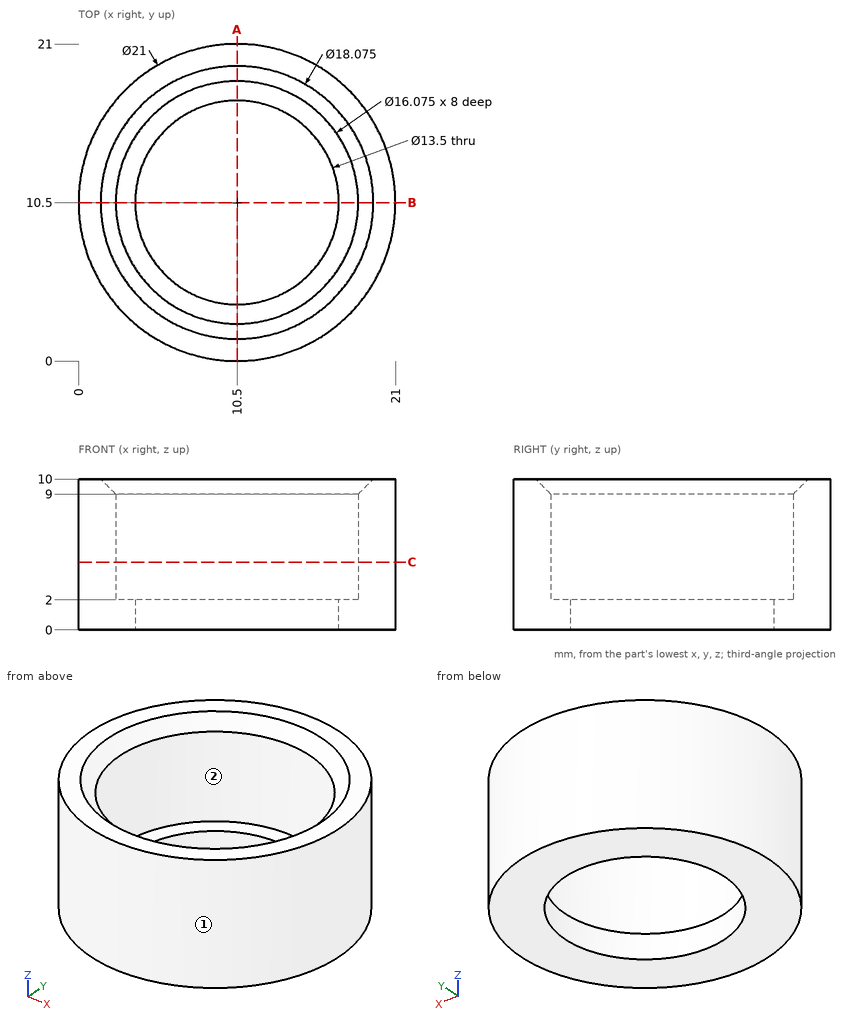
Geometry: see drawing. Coordinates: mm, zero at the bounding-box minimum. A direction names the side the tool comes from. Give positions to 0.01 mm unless a question says otherwise; leave off trailing zeros. Loops run counter-clockwise (first coordinate to the right, second up) from the corner with the lowest first, then second, coordinate; pieces in that order, holes last. Notation, with made-up numbers: (-25, -13) -> (15, -13) arc R13 ccw to (15, 5) -> close; hole circle Ø5 at (89.5, 78). An arc over 180 degrees is marked (long way). Use CSV: the item, a comma, the result in double quotes.
(1) Access query for the marked faces 1 and 2. Directions: +Z, -Z, +X, -X, +Y, -Y. A direction counts if a zero-diameter tool reaches every point of the face in a straight line with its end or side. Return the directions, or none.
From the geometry:
face 1,"+Z, -Z"
face 2,"+Z"
(2) First-contact query: P1, Ø1.5, axis at y = 15, z = 5.5, coming from the -X side; P2, Ø11, axis at x = 10.5, y = 10.5, coming from the -Z side; P3, Ø1, axis at x = 8.5, z = 2.5, coming from the +Y side; P4, Ø4, axis at x = 19, z = 5.5, coming from the -Y side. Flat tips, straight axial feed; report the tip coordinate or a pass-through.
From the geometry:
P1,"x = 0.69"
P2,"through"
P3,"y = 20.89"
P4,"y = 2.25"
(3) Cut plane A-A (x = 10.5). Output: boundary loops of the cut face in (y, z), plus the area to 3 significant figures.
From the geometry:
outline,"(0, 0) -> (3.75, 0) -> (3.75, 2) -> (2.46, 2) -> (2.46, 9) -> (1.46, 10) -> (0, 10) -> close; (17.25, 0) -> (21, 0) -> (21, 10) -> (19.54, 10) -> (18.54, 9) -> (18.54, 2) -> (17.25, 2) -> close"
area,"53.4 mm^2"
(4) Ray query, line 1 along Y through (x, z) = (10.5, 1.25); line 2 along Y through (x, z) = (10.5, 5.25); line 3 along X through (y, z) = (12.5, 5). Return the intervals inside material, ascending. Write a range as [from, to].
From the geometry:
line 1,"[0, 3.75], [17.25, 21]"
line 2,"[0, 2.46], [18.54, 21]"
line 3,"[0.19, 2.72], [18.28, 20.81]"
(5) Cut plane C-C (z = 4.5). Output: boundary loops of the cut face in (x, y) (1 decimal), plus the area to 3 significant figures.
From the geometry:
outline,"circle Ø21 at (10.5, 10.5); hole circle Ø16.1 at (10.5, 10.5)"
area,"143 mm^2"
